Can you work these out from the model? Positions are in its coordinate system, mm. Give positions to 0.01 mm unless a question says otherwise; leave off trailing zeros. Loops run counter-clockwise (first coordinate to the right, second up) from the corner with the lowest first, then second, coordinate; pieces in that order, holes last. Notation, with made-up numbers: (10.25, 67.5) -> (45.25, 67.5) arc R13 ccw to (45.25, 88.5) -> close; hole circle Ø3 at (43.5, 82). An arc over 180 degrees is marked (long way). Use CSV: the item, a comma, the result in double quotes.
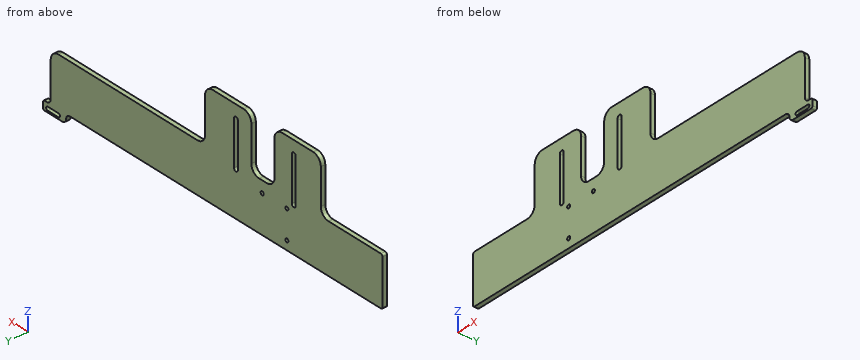
from build123d import *

# Parameters (mm, degrees)
SKETCH1_R           = 2
BOSS_EXTRUDE1_DEPTH = 5
SKETCH2_W           = 30
SKETCH2_H           = 10
BOSS_EXTRUDE2_DEPTH = 5
CUT_EXTRUDE1_DEPTH  = 315.880929877
FILLET1_R           = 5
SKETCH4_W           = 60
SKETCH4_H           = 60
BOSS_EXTRUDE3_DEPTH = 5
FILLET2_R           = 10
FILLET3_R           = 10
FILLET4_R           = 2
FILLET5_R           = 2
FILLET6_R           = 10
CUT_EXTRUDE2_DEPTH  = 331.681115276


with BuildPart() as part:
    # Sketch1 → Boss-Extrude1 (new body)
    with BuildSketch(Plane(origin=(0, 0, 0), x_dir=(1, 0, 0), z_dir=(0, 1, 0))):
        Polygon((0, 0), (-130, 0), (-130, -55), (300, -55), (300, 0), align=None)
        with Locations(Location((-6, -10, 0), (0, 0, 270))):
            Circle(SKETCH1_R, mode=Mode.SUBTRACT)
        with Locations(Location((-6, -42, 0), (0, 0, 90))):
            Circle(SKETCH1_R, mode=Mode.SUBTRACT)
        with Locations(Location((26, -42, 0), (0, 0, 270))):
            Circle(SKETCH1_R, mode=Mode.SUBTRACT)
    extrude(amount=BOSS_EXTRUDE1_DEPTH)

    # Sketch2 → Boss-Extrude2 (add)
    with BuildSketch(Plane(origin=(0, 5, 0), x_dir=(1, 0, 0), z_dir=(0, 1, 0))):
        with Locations((295, 5)):
            Rectangle(SKETCH2_W, SKETCH2_H)
    extrude(amount=-BOSS_EXTRUDE2_DEPTH)

    # Sketch3 → Cut-Extrude1 (cut, through all)
    with BuildSketch(Plane(origin=(0, 5, 0), x_dir=(1, 0, 0), z_dir=(0, 1, 0))):
        with BuildLine():
            Line((290, 8), (304, 8))
            ThreePointArc((304, 8), (306, 6), (304, 4))
            Line((304, 4), (290, 4))
            ThreePointArc((290, 4), (288, 6), (290, 8))
        make_face()
    extrude(amount=-CUT_EXTRUDE1_DEPTH, mode=Mode.SUBTRACT)

    # Fillet1
    fillet1_edges = [part.edges().sort_by_distance(p)[0] for p in [
        (300, 2.5, 0),
        (280, 2.5, -10),
        (280, 2.5, 0),
    ]]
    fillet(fillet1_edges, radius=FILLET1_R - 0.0001)  # a hair under: the kernel refuses the full size

    # Sketch4 → Boss-Extrude3 (add)
    with BuildSketch(Plane(origin=(0, 5, 0), x_dir=(1, 0, 0), z_dir=(0, 1, 0))):
        with Locations((70, -85)):
            Rectangle(SKETCH4_W, SKETCH4_H)
        with Locations((-20, -85)):
            Rectangle(SKETCH4_W, SKETCH4_H)
    extrude(amount=-BOSS_EXTRUDE3_DEPTH)

    # Fillet2
    fillet2_edges = [part.edges().sort_by_distance(p)[0] for p in [
        (40, 2.5, 55),
        (100, 2.5, 55),
        (100, 2.5, 115),
        (40, 2.5, 115),
    ]]
    fillet(fillet2_edges, radius=FILLET2_R)

    # Fillet3
    fillet3_edges = [part.edges().sort_by_distance(p)[0] for p in [
        (300, 2.5, 55),
    ]]
    fillet(fillet3_edges, radius=FILLET3_R)

    # Fillet4
    fillet4_edges = [part.edges().sort_by_distance(p)[0] for p in [
        (310, 2.5, -10),
        (310, 2.5, 0),
    ]]
    fillet(fillet4_edges, radius=FILLET4_R)

    # Fillet5
    fillet5_edges = [part.edges().sort_by_distance(p)[0] for p in [
        (-130, 2.5, 55),
        (-130, 2.5, 0),
    ]]
    fillet(fillet5_edges, radius=FILLET5_R)

    # Fillet6
    fillet6_edges = [part.edges().sort_by_distance(p)[0] for p in [
        (10, 2.5, 55),
        (10, 2.5, 115),
        (-50, 2.5, 115),
        (-50, 2.5, 55),
    ]]
    fillet(fillet6_edges, radius=FILLET6_R)

    # Sketch6 → Cut-Extrude2 (cut, through all)
    with BuildSketch(Plane(origin=(0, 5, 0), x_dir=(1, 0, 0), z_dir=(0, 1, 0))):
        with BuildLine():
            Line((-17.5, -100), (-17.5, -50))
            ThreePointArc((-17.5, -50), (-15, -47.5), (-12.5, -50))
            Line((-12.5, -50), (-12.5, -100))
            ThreePointArc((-12.5, -100), (-15, -102.5), (-17.5, -100))
        make_face()
        with BuildLine():
            Line((57.5, -100), (57.5, -50))
            ThreePointArc((57.5, -50), (60, -47.5), (62.5, -50))
            Line((62.5, -50), (62.5, -100))
            ThreePointArc((62.5, -100), (60, -102.5), (57.5, -100))
        make_face()
    extrude(amount=-CUT_EXTRUDE2_DEPTH, mode=Mode.SUBTRACT)


solid = part.part
(1) If we section it at D-D, the plane z = 25.5: Write out the boundary of the cut face in (x, y).
Answer sheet:
outline,"(-130, 0) -> (300, 0) -> (300, 5) -> (-130, 5) -> close"
(2) If we section it at C-C, the plane y = 1.95: Give the number of separate pieces and of enclosed holes in the cut face, then the cut area to 3 significant figures.
Answer sheet:
separate pieces,"1"
enclosed holes,"6"
area,"30,500 mm2"
(3) If we section it at B-B, the plane x = 185: Write out the boundary of the cut face in (y, z).
Answer sheet:
outline,"(0, 0) -> (5, 0) -> (5, 55) -> (0, 55) -> close"
(4) If we section it at A-A, the plane z = 95: Write out the boundary of the cut face in (x, y), then the cut area to 3 significant figures.
Answer sheet:
outline,"(-50, 0) -> (-17.5, 0) -> (-17.5, 5) -> (-50, 5) -> close; (-12.5, 0) -> (10, 0) -> (10, 5) -> (-12.5, 5) -> close; (40, 0) -> (57.5, 0) -> (57.5, 5) -> (40, 5) -> close; (62.5, 0) -> (100, 0) -> (100, 5) -> (62.5, 5) -> close"
area,"550 mm2"
(5) If I drill on L1, parallel to X at y = 1.8, z = 42; L2, parallel to X at y = 2, z = 72.5; L3, parallel to X at y = 2.55, z = 10, over which ranges is the centre line in solid material (lowest first)? Write a range as from..to.
Answer sheet:
L1,"x = -130..-8, -4..24, 28..300"
L2,"x = -50..-17.5, -12.5..10, 40..57.5, 62.5..100"
L3,"x = -130..-8, -4..300"
(6) Will these pins go through, and if not, where does the flat tip stop? pin 1 Ø1.5 at (x, y) = (-24, 3) entering from -Z; pin 2 Ø1.5 at (y, z) = (3.5, 21) entering from +X; pin 3 Ø1 at (x, z) = (-30, 47.5) entering from -Y; pin 4 Ø2.5 at (x, z) = (26, 42) entering from -Y (3 decimals).
Answer sheet:
pin 1,"stops at z = 0"
pin 2,"stops at x = 300"
pin 3,"stops at y = 0"
pin 4,"passes through"
